Input: part model. Units: mm. Frame: model coordinates. Round coordinates to 2 decimals unless told otherwise and drop trailing zeros. Loops run counter-clockwise (first coordinate to the right, second up) from the corner with the lowest first, then second, coordinate; pieces in that order, holes last. Notation, with made-up numbers: (17, 64.5) -> (53, 64.5) arc R32 ccw to (53, 90.5) -> close; hole circle Ø1 at (51, -27.75). An arc over 180 degrees is marked (long way). Answer in a Markdown table with one row per item. Add a question column.
Q1. Section A-A, the plane y = 27.5. Output: boundary loops of the cut face in (x, z), and give its area (3 significant figures).
Q2. Ray query, L1, parallel to X at y = 41.5, z = 2.5; L2, parallel to Y at x = 34.5, z = 10; L3, parallel to Y at x = 35, z = 14. Return the intervals inside material, ascending. Write a range as from..to.
Q3. Pin query (flat end, axial travel): pin 1 (5 mm diameter, centred on y = 59, z = 6.5, fed in from +X); pin 2 (7 mm diameter, centred on x = 32.43, y = 40.74, fed in from -Z); pin 3 (2 mm diameter, centred on y = -35.5, z = 3.5, fed in from +X); pin 4 (1 mm diameter, centred on y = -3, z = 9.5, fed in from -X). Return the tip coordinate at first contact, or that it passes through.
```python
from build123d import *

# Parameters (mm, degrees)
BOSS_EXTRU_1_DEPTH                                 = 15
CHAMBRAGE_POUR_VIS_T_TE_HEXAGONALE_M81_D           = 9
CHAMBRAGE_POUR_VIS_T_TE_HEXAGONALE_M81_CBORE_D     = 15
CHAMBRAGE_POUR_VIS_T_TE_HEXAGONALE_M81_CBORE_DEPTH = 8.6
TAP_DRILL_FOR_M5_TAP1_D                            = 4.2
TAP_DRILL_FOR_M5_TAP1_DEPTH                        = 13
TAP_DRILL_FOR_M5_TAP1_TIP                          = 1.2618073
SKETCH25_W                                         = 14
SKETCH25_H                                         = 15
CUT_EXTRUDE6_DEPTH                                 = 16
CONG_1_R                                           = 6
SKETCH11_R                                         = 8.5
CUT_EXTRUDE1_DEPTH                                 = 16
SKETCH12_R                                         = 11
CUT_EXTRUDE2_DEPTH                                 = 11
SKETCH13_W                                         = 24
SKETCH13_H                                         = 24
CUT_EXTRUDE3_DEPTH                                 = 16
FILLET1_R                                          = 6
CUT_EXTRUDE4_DEPTH                                 = 6
FILLET3_R                                          = 14
TAP_DRILL_FOR_M3_TAP1_D                            = 2.5
CHAMFER1_SIZE                                      = 0.5
TAP_DRILL_FOR_M3_TAP2_D                            = 2.5
TAP_DRILL_FOR_M3_TAP3_D                            = 2.5


with BuildPart() as part:
    # Esquisse1 → Boss.-Extru.1 (new body)
    with BuildSketch(Plane.XY):
        Polygon((-21.072673536, 123.242590707), (54.927326464, 123.242590707), (54.927326464, 18.242590707), (130.927326464, 18.242590707), (130.927326464, -26.757409293), (115.927326464, -26.757409293), (-4.072673536, -146.757409293), (-169.072673536, -146.757409293), (-169.072673536, -76.757409293), (-139.072673536, -46.757409293), (-88.072673536, -46.757409293), (-41.072673536, 0.242590707), (-41.072673536, 103.242590707), align=None)
    extrude(amount=BOSS_EXTRU_1_DEPTH)

    # Chambrage pour vis à tête hexagonale M81 (through all)
    with Locations(Plane(origin=(0, 0, 0), x_dir=(-1, 0, 0), z_dir=(0, 0, -1))):
        with Locations((72.572673536, -78.257409293), (117.572673536, -78.257409293), (72.572673536, -135.257409293), (117.572673536, -135.257409293), (-32.427326464, 85.742590707), (-32.427326464, 40.742590707), (-32.427326464, -4.257409293), (-77.427326464, -4.257409293), (12.572673536, 40.742590707)):
            CounterBoreHole(CHAMBRAGE_POUR_VIS_T_TE_HEXAGONALE_M81_D / 2, CHAMBRAGE_POUR_VIS_T_TE_HEXAGONALE_M81_CBORE_D / 2, CHAMBRAGE_POUR_VIS_T_TE_HEXAGONALE_M81_CBORE_DEPTH)

    # Tap Drill for M5 Tap1
    with Locations(Plane(origin=(0, -146.757409293, 0), x_dir=(-1, 0, 0), z_dir=(0, -1, 0))):
        with Locations((13.072673536, -7.5)):
            Hole(TAP_DRILL_FOR_M5_TAP1_D / 2, depth=TAP_DRILL_FOR_M5_TAP1_DEPTH)
            with Locations((0, 0, -(TAP_DRILL_FOR_M5_TAP1_DEPTH + TAP_DRILL_FOR_M5_TAP1_TIP / 2))):  # 118° drill point
                Cone(0, TAP_DRILL_FOR_M5_TAP1_D / 2, TAP_DRILL_FOR_M5_TAP1_TIP, mode=Mode.SUBTRACT)

    # Sketch25 → Cut-Extrude6 (cut, through all)
    with BuildSketch(Plane(origin=(0, 0, 0), x_dir=(-1, 0, 0), z_dir=(0, 0, -1))):
        with Locations((95.072673536, -54.257409293)):
            Rectangle(SKETCH25_W, SKETCH25_H)
    extrude(amount=-CUT_EXTRUDE6_DEPTH, mode=Mode.SUBTRACT)

    # Congé1
    cong_1_edges = [part.edges().sort_by_distance(p)[0] for p in [
        (-88.072673536, -61.757409293, 7.5),
        (-102.072673536, -46.757409293, 7.5),
        (-102.072673536, -61.757409293, 7.5),
        (54.927326464, 18.242590707, 7.5),
        (130.927326464, 18.242590707, 7.5),
        (130.927326464, -26.757409293, 7.5),
        (115.927326464, -26.757409293, 7.5),
        (-4.072673536, -146.757409293, 7.5),
        (-169.072673536, -76.757409293, 7.5),
        (-139.072673536, -46.757409293, 7.5),
        (-88.072673536, -46.757409293, 7.5),
        (-41.072673536, 0.242590707, 7.5),
        (-41.072673536, 103.242590707, 7.5),
        (-21.072673536, 123.242590707, 7.5),
        (54.927326464, 123.242590707, 7.5),
    ]]
    fillet(cong_1_edges, radius=CONG_1_R)

    # Sketch11 → Cut-Extrude1 (cut, through all)
    with BuildSketch(Plane(origin=(0, 0, 0), x_dir=(-1, 0, 0), z_dir=(0, 0, -1))):
        with Locations((155.072673536, -132.757409293)):
            Circle(SKETCH11_R)
    extrude(amount=-CUT_EXTRUDE1_DEPTH, mode=Mode.SUBTRACT)

    # Sketch12 → Cut-Extrude2 (cut)
    with BuildSketch(Plane(origin=(0, 0, 0), x_dir=(-1, 0, 0), z_dir=(0, 0, -1))):
        with Locations((155.072673536, -132.757409293)):
            Circle(SKETCH12_R)
    extrude(amount=-CUT_EXTRUDE2_DEPTH, mode=Mode.SUBTRACT)

    # Sketch13 → Cut-Extrude3 (cut, through all)
    with BuildSketch(Plane(origin=(0, 0, 0), x_dir=(-1, 0, 0), z_dir=(0, 0, -1))):
        with Locations((48.572673536, -36.757409293)):
            Rectangle(SKETCH13_W, SKETCH13_H)
    extrude(amount=-CUT_EXTRUDE3_DEPTH, mode=Mode.SUBTRACT)

    # Fillet1
    fillet1_edges = [part.edges().sort_by_distance(p)[0] for p in [
        (-36.572673536, -48.757409293, 7.5),
        (-36.572673536, -24.757409293, 7.5),
        (-60.572673536, -24.757409293, 7.5),
        (-60.572673536, -48.757409293, 7.5),
    ]]
    fillet(fillet1_edges, radius=FILLET1_R)

    # Sketch14 → Cut-Extrude4 (cut)
    with BuildSketch(Plane(origin=(0, 0, 0), x_dir=(-1, 0, 0), z_dir=(0, 0, -1))):
        with BuildLine():
            Line((53.794093198, -18.414240629), (59.625660306, -27.52208478))
            ThreePointArc((59.625660306, -27.52208478), (60.33105528, -29.071870895), (60.572673536, -30.757409293))
            Line((60.572673536, -30.757409293), (60.572673536, -42.757409293))
            ThreePointArc((60.572673536, -42.757409293), (60.33105528, -44.442947691), (59.625660306, -45.992733806))
            Line((59.625660306, -45.992733806), (53.794093198, -55.100577956))
            ThreePointArc((53.794093198, -55.100577956), (48.572673536, -57.957409293), (43.351253874, -55.100577956))
            Line((43.351253874, -55.100577956), (37.519686767, -45.992733806))
            ThreePointArc((37.519686767, -45.992733806), (36.814291792, -44.442947691), (36.572673536, -42.757409293))
            Line((36.572673536, -42.757409293), (36.572673536, -30.757409293))
            ThreePointArc((36.572673536, -30.757409293), (36.814291792, -29.071870895), (37.519686767, -27.52208478))
            Line((37.519686767, -27.52208478), (43.351253874, -18.414240629))
            ThreePointArc((43.351253874, -18.414240629), (48.572673536, -15.557409293), (53.794093198, -18.414240629))
        make_face()
    extrude(amount=-CUT_EXTRUDE4_DEPTH, mode=Mode.SUBTRACT)

    # Fillet3
    fillet3_edges = [part.edges().sort_by_distance(p)[0] for p in [
        (-169.072673536, -146.757409293, 7.5),
    ]]
    fillet(fillet3_edges, radius=FILLET3_R)

    # Tap Drill for M3 Tap1 (through all)
    with Locations(Plane(origin=(0, 0, 6), x_dir=(-1, 0, 0), z_dir=(0, 0, -1))):
        with Locations((48.572673536, -21.757409293), (48.572673536, -51.757409293)):
            Hole(TAP_DRILL_FOR_M3_TAP1_D / 2)

    # Chamfer1
    chamfer1_edges = [part.edges().sort_by_distance(p)[0] for p in [
        (-102.072673536, -54.257409293, 0),
        (-95.072673536, -61.757409293, 0),
        (-88.072673536, -52.50004998, 0),
        (-122.330032849, -46.757409293, 0),
        (-64.572673536, -23.257409293, 0),
        (-41.072673536, 51.742590707, 0),
        (-31.072673536, 113.242590707, 0),
        (15.169967151, 123.242590707, 0),
        (54.927326464, 70.742590707, 0),
        (92.927326464, 18.242590707, 0),
        (130.927326464, -4.257409293, 0),
        (121.669967151, -26.757409293, 0),
        (55.927326464, -86.757409293, 0),
        (-169.072673536, -106.00004998, 0),
        (-154.072673536, -61.757409293, 0),
        (53.169967151, 121.485231394, 0),
        (-20.883492756, 122.785867902, 0),
        (-138.883492756, -47.214132098, 0),
        (-168.615950731, -76.946590073, 0),
        (-40.615950731, 103.053409927, 0),
        (129.169967151, 16.485231394, 0),
        (129.169967151, -25.00004998, 0),
        (-4.261854316, -146.300686488, 0),
        (-87.615950731, -46.946590073, 0),
        (-103.830032849, -48.514768606, 0),
        (-100.315314223, -60.00004998, 0),
        (-89.830032849, -60.00004998, 0),
        (116.116507244, -27.214132098, 0),
        (-41.529396341, 0.431771487, 0),
        (56.684685777, 19.99995002, 0),
        (-144.072673536, -132.757409293, 0),
        (-60.572673536, -36.757409293, 0),
        (-36.572673536, -36.757409293, 0),
        (-60.33105528, -44.442947691, 0),
        (-36.814291792, -29.071870895, 0),
        (-60.33105528, -29.071870895, 0),
        (-36.814291792, -44.442947691, 0),
        (-56.709876752, -50.546655881, 0),
        (-40.43547032, -50.546655881, 0),
        (-48.572673536, -57.957409293, 0),
        (-40.43547032, -22.968162704, 0),
        (-56.709876752, -22.968162704, 0),
        (-48.572673536, -15.557409293, 0),
        (-80.815314223, -146.757409293, 0),
        (-164.972168473, -142.656904229, 0),
        (-5.072673536, 40.742590707, 0),
        (84.927326464, -4.257409293, 0),
        (39.927326464, -4.257409293, 0),
        (39.927326464, 40.742590707, 0),
        (39.927326464, 85.742590707, 0),
        (-110.072673536, -135.257409293, 0),
        (-65.072673536, -135.257409293, 0),
        (-110.072673536, -78.257409293, 0),
        (-65.072673536, -78.257409293, 0),
    ]]
    chamfer(chamfer1_edges, length=CHAMFER1_SIZE)

    # Tap Drill for M3 Tap2 (through all)
    with Locations(Plane(origin=(0, 0, 0), x_dir=(-1, 0, 0), z_dir=(0, 0, -1))):
        with Locations((-124.927326464, 12.242590707), (-124.927326464, -20.757409293), (-60.927326464, 12.242590707), (-60.927326464, -20.757409293)):
            Hole(TAP_DRILL_FOR_M3_TAP2_D / 2)

    # Tap Drill for M3 Tap3 (through all)
    with Locations(Plane.XY.offset(15)):
        with Locations((-111.072673536, -52.057409293), (-111.072673536, -62.457409293), (-79.072673536, -62.457409293), (-79.072673536, -52.057409293)):
            Hole(TAP_DRILL_FOR_M3_TAP3_D / 2)


solid = part.part
```
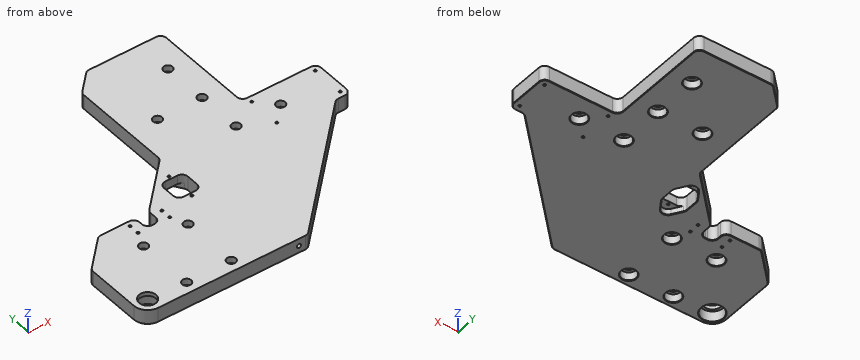
Answer block:
| question | item | result |
|---|---|---|
| 1 | outline | (-41.07, 0.5) -> (-40.57, 0) -> (54.43, 0) -> (54.93, 0.5) -> (54.93, 15) -> (-41.07, 15) -> close |
| 1 | area | 1,440 mm^2 |
| 2 | L1 | -41.07..-20.03, -5.11..24.97, 39.89..54.93 |
| 2 | L2 | -108.18..-8.25, -0.26..36.75, 44.74..81.75, 89.74..123.24 |
| 2 | L3 | -107.68..-7.95, -0.57..37.05, 44.43..82.05, 89.43..123.24 |
| 3 | pin 1 | x = 54.93 |
| 3 | pin 2 | through |
| 3 | pin 3 | x = 108.18 |
| 3 | pin 4 | x = -44.82 |
